Model file for the job. Use its own axes, mm. A direction names the side the tool comes from. Give positions to 0.01 mm unless a question says otherwise; leave off trailing zeros. Loops run counter-clockwise (first coordinate to the right, second up) from the corner with the lowest first, then second, coordinate; pieces in that order, holes last. Notation, with made-up numbers: M 59,-40 L 101,-40 A25 cw 101,-1 Z; hole C 72.25,63.5 d10. An arc over 180 degrees is marked long. Answer in a Markdown table with one row per item.
```python
from build123d import *

# Parameters (mm, degrees)
ESQUISSE1_W             = 135
ESQUISSE1_H             = 53
BOSS_EXTRU_1_DEPTH      = 3
ESQUISSE2_R             = 9
ENL_V_MAT_EXTRU_1_DEPTH = 4
ESQUISSE3_W             = 3
ESQUISSE3_H             = 33
BOSS_EXTRU_2_DEPTH      = 3
ESQUISSE4_W             = 3
ESQUISSE4_H             = 33
BOSS_EXTRU_3_DEPTH      = 3
ESQUISSE5_W             = 40
ESQUISSE5_H             = 3
BOSS_EXTRU_4_DEPTH      = 3.4
ESQUISSE6_W             = 40
ESQUISSE6_H             = 3
BOSS_EXTRU_5_DEPTH      = 3.4


with BuildPart() as part:
    # Esquisse1 → Boss.-Extru.1 (new body)
    with BuildSketch(Plane.XY):
        with Locations((-41.062592566, -45.035528327)):
            Rectangle(ESQUISSE1_W, ESQUISSE1_H)
    extrude(amount=BOSS_EXTRU_1_DEPTH)

    # Esquisse2 → Enlèv. mat.-Extru.1 (cut, through all)
    with BuildSketch(Plane(origin=(0, 0, 0), x_dir=(-1, 0, 0), z_dir=(0, 0, -1))):
        with Locations((0.403677713, -41.89919031)):
            Circle(ESQUISSE2_R)
    extrude(amount=-ENL_V_MAT_EXTRU_1_DEPTH, mode=Mode.SUBTRACT)

    # Esquisse3 → Boss.-Extru.2 (add)
    with BuildSketch(Plane(origin=(26.437407434, 0, 0), x_dir=(0, 0, -1), z_dir=(1, 0, 0))):
        with Locations((-1.5, -45.035528327)):
            Rectangle(ESQUISSE3_W, ESQUISSE3_H)
    extrude(amount=BOSS_EXTRU_2_DEPTH)

    # Esquisse4 → Boss.-Extru.3 (add)
    with BuildSketch(Plane.ZY.offset(108.562592566)):
        with Locations((1.5, -45.035528327)):
            Rectangle(ESQUISSE4_W, ESQUISSE4_H)
    extrude(amount=BOSS_EXTRU_3_DEPTH)

    # Esquisse5 → Boss.-Extru.4 (add)
    with BuildSketch(Plane(origin=(0, -18.535528327, 0), x_dir=(1, 0, 0), z_dir=(0, 1, 0))):
        with Locations((-73.562592566, -1.5)):
            Rectangle(ESQUISSE5_W, ESQUISSE5_H)
    extrude(amount=BOSS_EXTRU_4_DEPTH)

    # Esquisse6 → Boss.-Extru.5 (add)
    with BuildSketch(Plane(origin=(0, -18.535528327, 0), x_dir=(1, 0, 0), z_dir=(0, 1, 0))):
        with Locations((-8.562592566, -1.5)):
            Rectangle(ESQUISSE6_W, ESQUISSE6_H)
    extrude(amount=BOSS_EXTRU_5_DEPTH)


solid = part.part
```
Q1. Saw through at B-B (y = -47). Give the cut face in (x, z).
Reported:
| item | result |
|---|---|
| outline | M -111.56,0 L -7.82,0 L -7.82,3 L -111.56,3 Z; M 7.01,0 L 29.44,0 L 29.44,3 L 7.01,3 Z |
Q2. Saw through at D-D (x = 15.5). Give the cut face in (y, z).
Reported:
| item | result |
|---|---|
| outline | M -71.54,0 L -18.54,0 L -18.54,3 L -71.54,3 Z |
Q3. Drop flat-ended pins along their axis: pin 1 (0.9 mm diameter, centred on x = -101, z = 1.5, fed in from +Y); pin 2 (1.5 mm diameter, centred on y = -17, z = 1.5, fed in from +X); pin 3 (0.9 mm diameter, centred on y = -17.5, z = 1, fed in from -X). Give the stop position or say it passes through.
Reported:
| item | result |
|---|---|
| pin 1 | y = -18.54 |
| pin 2 | x = 11.44 |
| pin 3 | x = -93.56 |
Q4. 3-axis set-ups, long thin cutter, end or side, ignore diameter. For faces 1 (the face through (-110, -61.536, 1)), 2 (the face through (19, -18.536, 1)), 3 (the face through (-101, -18.536, 1)), 4 (the face through (26.437, -67, 1)), 5 (the face through (-28.563, -17, 2)): which of +Z, -Z, +X, -X, +Y, -Y reach the whole face in a straight line?
Reported:
| item | result |
|---|---|
| face 1 | +Z, -Z, -X, -Y |
| face 2 | +Z, -Z, +X, +Y |
| face 3 | +Z, -Z, -X, +Y |
| face 4 | +Z, -Z, +X, -Y |
| face 5 | +Z, -Z, +Y |
Q5. Saw through at A-A (x = 0). Give the cut face in (y, z), and give its area (3 significant figures).
Reported:
| item | result |
|---|---|
| outline | M -71.54,0 L -50.89,0 L -50.89,3 L -71.54,3 Z; M -32.91,0 L -15.14,0 L -15.14,3 L -32.91,3 Z |
| area | 115 mm² |
Q6. Probe probe 1 along Y at (x, z) = (-97, 1.45); probe 2 along Y at (x, z) = (-4, 2.8); probe 3 along X at (y, z) = (-46.5, 2.55). List the from-to ranges inside material, lowest first.
Reported:
| item | result |
|---|---|
| probe 1 | -71.54 to -18.54 |
| probe 2 | -71.54 to -50.15, -33.65 to -15.14 |
| probe 3 | -111.56 to -8.14, 7.33 to 29.44 |
Q7. Saw through at C-C (z = 2.55). Give the cut face in (x, y), and give its area (3 significant figures).
Reported:
| item | result |
|---|---|
| outline | M -111.56,-61.54 L -108.56,-61.54 L -108.56,-71.54 L 26.44,-71.54 L 26.44,-61.54 L 29.44,-61.54 L 29.44,-28.54 L 26.44,-28.54 L 26.44,-18.54 L 11.44,-18.54 L 11.44,-15.14 L -28.56,-15.14 L -28.56,-18.54 L -53.56,-18.54 L -53.56,-15.14 L -93.56,-15.14 L -93.56,-18.54 L -108.56,-18.54 L -108.56,-28.54 L -111.56,-28.54 Z; hole C -0.4,-41.9 d18 |
| area | 7,370 mm² |
Q8. Mould opens along X. For faces 6 (the face through (-42, -43, 0)), 7 (the face through (-53.563, -17, 2)), 8 (the face through (-93.563, -17, 2)) say: released by +X, released by -X, zero draft, split by the parting line, or undercut.
Reported:
| item | result |
|---|---|
| face 6 | zero draft |
| face 7 | undercut |
| face 8 | released by -X |
